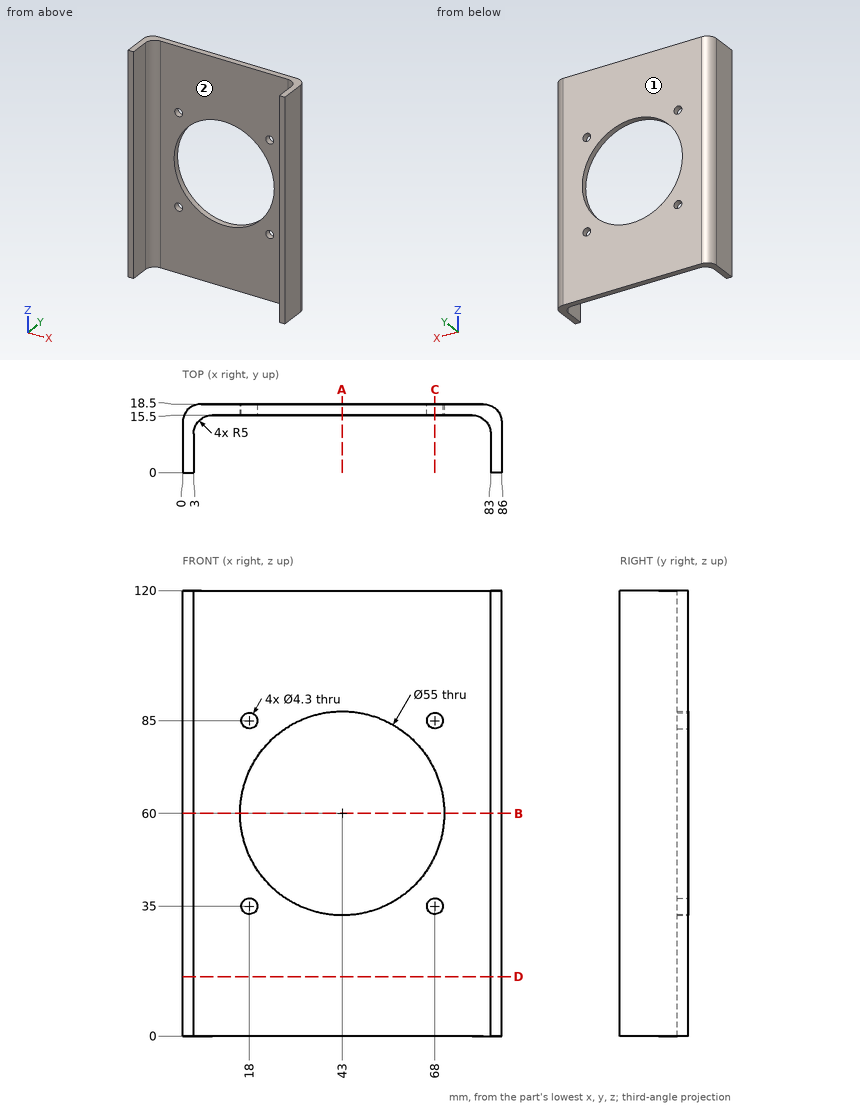
Verification items for this drawing (mm, ordinates from the low corner). A direction names the side the tool comes from. Round coordinates to 2 decimals unless told otherwise and drop trailing zeros. Loops run counter-clockwise (first coordinate to the right, second up) from the corner with the lowest first, then second, coordinate; pieces in that order, holes last. Notation, with made-up numbers: (33.5, 0.5) -> (48.5, 0.5) arc R16 ccw to (48.5, 22.5) -> close; hole circle Ø3 at (47, 55.5). An arc over 180 degrees is marked (long way). Answer in a Markdown table with one row per item.
Q1. Go/stop test with flat-tipped pins: P1, Ø10, axis at x = 76, z = 74.5, coming from the -Y side; P2, Ø5, axis at x = 18, z = 35, coming from the -Y side. Record where each tip stops, or that it passes through.
Data:
| item | result |
|---|---|
| P1 | stops at y = 14.5 |
| P2 | stops at y = 15.5 |
Q2. Sectioned sample at B-B on z = 60. Enter the section's corners in (x, y), then the cut area to 3 significant figures.
Data:
| item | result |
|---|---|
| outline | (0, 0) -> (3, 0) -> (3, 10.5) arc R5 cw to (8, 15.5) -> (15.5, 15.5) -> (15.5, 18.5) -> (5, 18.5) arc R5 ccw to (0, 13.5) -> close; (70.5, 15.5) -> (78, 15.5) arc R5 cw to (83, 10.5) -> (83, 0) -> (86, 0) -> (86, 13.5) arc R5 ccw to (81, 18.5) -> (70.5, 18.5) -> close |
| area | 186 mm^2 |
Q3. Thickness scan on L1, parallel to X at y = 16.35, z = 85; L2, parallel to X at y = 7.5, z = 74; L3, parallel to Z at x = 68, y = 16.65. Record the ranges inside material, lowest first.
Data:
| item | result |
|---|---|
| L1 | x = 0.89 to 15.85, 20.15 to 31.54, 54.46 to 65.85, 70.15 to 85.11 |
| L2 | x = 0 to 3, 83 to 86 |
| L3 | z = 0 to 32.85, 37.15 to 48.54, 71.46 to 82.85, 87.15 to 120 |
Q4. Sectioned sample at C-C on x = 68. Enter the section's corners in (y, z).
Data:
| item | result |
|---|---|
| outline | (15.5, 0) -> (18.5, 0) -> (18.5, 32.85) -> (15.5, 32.85) -> close; (15.5, 37.15) -> (18.5, 37.15) -> (18.5, 48.54) -> (15.5, 48.54) -> close; (15.5, 71.46) -> (18.5, 71.46) -> (18.5, 82.85) -> (15.5, 82.85) -> close; (15.5, 87.15) -> (18.5, 87.15) -> (18.5, 120) -> (15.5, 120) -> close |
Q5. Set-up check for the marked faces 1 and 2: record each of +Z, -Z, +X, -X, +Y, -Y from which the full face is reachable in a straight line by a thin tool's end or side.
Data:
| item | result |
|---|---|
| face 1 | +Z, -Z, +X, -X, +Y |
| face 2 | +Z, -Z, -Y |
Q6. Sectioned sample at A-A on x = 43. Enter the section's corners in (y, z).
Data:
| item | result |
|---|---|
| outline | (15.5, 0) -> (18.5, 0) -> (18.5, 32.5) -> (15.5, 32.5) -> close; (15.5, 87.5) -> (18.5, 87.5) -> (18.5, 120) -> (15.5, 120) -> close |
Q7. Sectioned sample at D-D on z = 16. Enter the section's corners in (x, y).
Data:
| item | result |
|---|---|
| outline | (0, 0) -> (3, 0) -> (3, 10.5) arc R5 cw to (8, 15.5) -> (78, 15.5) arc R5 cw to (83, 10.5) -> (83, 0) -> (86, 0) -> (86, 13.5) arc R5 ccw to (81, 18.5) -> (5, 18.5) arc R5 ccw to (0, 13.5) -> close |
